Part model, mm, in its own coordinate system. Give positions to 0.01 mm unless a question says otherwise; leave off trailing zeros. Write each loop counter-clockwise with the first axis right and the second up, starting at its lowest first coordinate (ties: lowest second). Pieces come first, ordered by that corner, then holes.
Autodesk Inventor part; units mm, degrees
ref_plane "YZ Plane" through (0, 0, 0) normal (1, 0, 0) x (0, 1, 0)
ref_plane "XZ Plane" through (0, 0, 0) normal (0, 1, 0) x (-1, 0, 0)
ref_plane "XY Plane" through (0, 0, 0) normal (0, 0, 1) x (1, 0, 0)
sketch "スケッチ1" plane through (0, 0, 0) normal (0, 0, 1) x (1, 0, 0)
  line L0 (-100, -100) -> (100, -100)
  line L1 (100, -100) -> (100, 100)
  line L2 (100, 100) -> (-100, 100)
  line L3 (-100, 100) -> (-100, -100)
  line L4 (-100, -100) -> (100, 100) construction
  line L5 (100, -100) -> (-100, 100) construction
  point P0 (0, 0)
  dimension "d0" = 200
  dimension "d1" = 200
extrude "押し出し1" add sketch "スケッチ1" along normal blind 1.5
fillet "フィレット1" radius 40 2 edges at (-100, -100, 0.75) (100, -100, 0.75)
sketch "スケッチ3" plane through (0, 0, 0) normal (0, 0, -1) x (-1, 0, 0)
  point P0 (0, 0)
sketch "スケッチ4" plane through (0, 0, 1.5) normal (0, 0, 1) x (1, 0, 0)
  line L0 (100, -60) -> (100, 100)
  line L1 (100, 100) -> (50, 100)
  line L2 (50, 100) -> (50, 50)
  line L3 (50, 50) -> (100, 50)
  line L4 (100, 50) -> (100, 100)
  line L5 (100, 100) -> (-100, 100)
  line L6 (-100, 100) -> (-50, 100)
  line L7 (-50, 100) -> (-50, 50)
  line L8 (-50, 50) -> (-100, 50)
  line L9 (-100, 50) -> (-100, 100)
  point P0 (0, 0)
  dimension "d13" = 50
  dimension "d14" = 50
  dimension "d15" = 50
  dimension "d16" = 50
extrude "押し出し2" cut sketch "スケッチ4" against normal through all
sketch "スケッチ5" plane through (0, 0, 1.5) normal (0, 0, 1) x (1, 0, 0)
  line L0 (-100, 50) -> (-100, -60)
  line L1 (-88, -64) -> (-100, -64)
  line L2 (-100, -64) -> (-100, -16)
  line L3 (-100, -16) -> (-88, -16)
  line L4 (-88, -16) -> (-88, -64)
  line L5 (-60, -100) -> (60, -100)
  line L6 (100, -60) -> (100, 50)
  line L7 (88, -64) -> (100, -64)
  line L8 (100, -64) -> (100, -16)
  line L9 (100, -16) -> (88, -16)
  line L10 (88, -16) -> (88, -64)
  point P0 (0, 0)
  dimension "d19" = 12
  dimension "d20" = 36
  dimension "d21" = 48
  dimension "d24" = 36
  dimension "d25" = 48
  dimension "d26" = 12
extrude "押し出し3" cut sketch "スケッチ5" against normal through all
fillet "フィレット2" radius 2 8 edges at (99.7995, -64, 0.75) (88, -64, 0.75) (100, -16, 0.75) (88, -16, 0.75) (-100, -16, 0.75) (-88, -16, 0.75) (-99.7995, -64, 0.75) (-88, -64, 0.75)
sketch "スケッチ6" plane through (0, 0, 1.5) normal (0, 0, 1) x (1, 0, 0)
  point P0 (0, 0)
fillet "フィレット3" radius 10 6 edges at (50, 100, 0.75) (50, 50, 0.75) (100, 50, 0.75) (-100, 50, 0.75) (-50, 50, 0.75) (-50, 100, 0.75)
sketch "スケッチ7" plane through (0, 0, 1.5) normal (0, 0, 1) x (1, 0, 0)
  line L0 (-100, 40) -> (-100, -14)
  line L1 (-60, 50) -> (-90, 50)
  line L2 (90, 50) -> (60, 50)
  line L3 (100, -14) -> (100, 40)
  line L4 (40, 100) -> (-40, 100)
  line L5 (50, 60) -> (50, 90)
  line L6 (-50, 90) -> (-50, 60)
  point P0 (0, 0)
  point P1 (-90, 40)
  point P2 (90, 40)
  point P3 (-40, 90)
  point P4 (40, 90)
  point P5 (40, 0)
  point P6 (-40, 0)
  dimension "d29" = 10
  dimension "d30" = 10
  dimension "d31" = 10
  dimension "d32" = 10
  dimension "d33" = 10
  dimension "d34" = 10
  dimension "d35" = 10
  dimension "d36" = 10
  dimension "d37" = 50
  dimension "d38" = 50
hole "穴2" at (-90, 40, 1.5) at (90, 40, 1.5) at (-40, 90, 1.5) at (40, 90, 1.5) at (40, 0, 1.5) at (-40, 0, 1.5) direction (0, 0, -1) diameter 3.5 end through all
sketch "スケッチ8" plane through (0, 0, 1.5) normal (0, 0, 1) x (1, 0, 0)
  circle A0 centre (68.5, -55.9) radius 2.15
  circle A1 centre (49.5, -55.9) radius 2.15
  circle A2 centre (49.5, -24.1) radius 2.15
  circle A3 centre (68.5, -24.1) radius 2.15
  circle A4 centre (-49.5, -24.1) radius 2.15
  circle A5 centre (-68.5, -24.1) radius 2.15
  circle A6 centre (-49.5, -55.9) radius 2.15
  circle A7 centre (-68.5, -55.9) radius 2.15
  point P0 (0, 0)
hole "穴3" at (49.5, -55.9, 1.5) at (68.5, -55.9, 1.5) at (49.5, -24.1, 1.5) at (68.5, -24.1, 1.5) at (-49.5, -55.9, 1.5) at (-49.5, -24.1, 1.5) at (-68.5, -24.1, 1.5) at (-68.5, -55.9, 1.5) direction (0, 0, -1) diameter 3.5 end through all
sketch "スケッチ9" plane through (0, 0, 0) normal (0, 0, -1) x (-1, 0, 0)
  line L0 (0, 0) -> (0, -75.963)
  line L1 (60, -100) -> (-60, -100)
  point P0 (8, -44)
  point P1 (-8, -44)
  point P2 (8, -30)
  point P3 (-8, -30)
  dimension "d53" = 14
  dimension "d54" = 16
  dimension "d62" = 56
hole "穴4" at (-8, -44, 0) at (8, -44, 0) at (-8, -30, 0) at (8, -30, 0) direction (0, 0, 1) diameter 3.5 end through all
sketch "スケッチ10" plane through (0, 0, 0) normal (0, 0, -1) x (-1, 0, 0)
  line L0 (0, 0) -> (0, -140.1942)
  line L1 (60, -100) -> (-60, -100)
  point P0 (-10, -97)
  point P1 (10, -97)
  point P2 (-30, -97)
  point P3 (-50, -97)
  point P4 (30, -97)
  point P5 (50, -97)
  dimension "d63" = 10
  dimension "d64" = 3
  dimension "d65" = 20
  dimension "d66" = 20
hole "穴5" at (10, -97, 0) at (-10, -97, 0) at (30, -97, 0) at (50, -97, 0) at (-30, -97, 0) at (-50, -97, 0) direction (0, 0, 1) diameter 3.5 end through all
sketch "スケッチ11" plane through (0, 0, 0) normal (0, 0, -1) x (-1, 0, 0)
  circle A0 centre (-9.7395, 8) radius 2.25
  circle A1 centre (-9.7395, 18) radius 2.25
  circle A2 centre (9.7395, 18) radius 2.25
  circle A3 centre (9.7395, 8) radius 2.25
  arc A4 (15, 20) -> (13, 22) centre (13, 20) ccw
  line L0 (14, 4) -> (-14, 4)
  arc A5 (-13, 22) -> (-15, 20) centre (-13, 20) ccw
  line L1 (-13, 22) -> (13, 22)
  line L2 (15, 20) -> (15, 3)
  arc A6 (15, 3) -> (14, 4) centre (14, 3) ccw
  arc A7 (-14, 4) -> (-15, 3) centre (-14, 3) ccw
  line L3 (-15, 3) -> (-15, 20)
  point P0 (0, 0)
  point P1 (15, 4)
  point P2 (-15, 4)
hole "穴6" at (9.7395, 8, 0) at (-9.7395, 8, 0) at (-9.7395, 18, 0) at (9.7395, 18, 0) direction (0, 0, 1) diameter 3.5 end through all
properties part number "台車土台" material "アルミニウム 6061"
1) Saw through at A-A, the plane z = 0.5. Count the separate pieces of the cut face and the enclosed holes in it, then the cut area to 3 significant figures.
Answers follow:
separate pieces: 1
enclosed holes: 28
area: 32,800 mm2
2) Pin check, flat tips, straight feed: pin 1 Ø4 at (x, y) = (-40, 90) entering from -Z; pin 2 Ø2 at (x, y) = (49.5, -55.9) entering from -Z; pin 3 Ø0.8 at (y, z) = (-36, 1) entering from +X. Stop position of each tip, or through.
Answers follow:
pin 1: stops at z = 0
pin 2: passes through
pin 3: stops at x = 88
3) Saw through at B-B, the plane y = 56.5. Write the cut outline in (x, z), then the cut area to 3 significant figures.
Answers follow:
outline: (-50.63, 0) - (50.63, 0) - (50.63, 1.5) - (-50.63, 1.5) - close
area: 152 mm2
4) Wall check: L1, parallel to X at y = 90, z = 0.9; L2, parallel to X at y = -55.9, z = 0.4; L3, parallel to X at y = 40, z = 0.7. Give the ranges that are in metal, low to high.
Answers follow:
L1: x = -50 to -41.75, -38.25 to 38.25, 41.75 to 50
L2: x = -88 to -70.25, -66.75 to -51.25, -47.75 to 47.75, 51.25 to 66.75, 70.25 to 88
L3: x = -100 to -91.75, -88.25 to 88.25, 91.75 to 100
